```python
from build123d import *

# Parameters (mm, degrees)
F0_W     = 50
F0_H     = 50
F0_W_2   = 46
F0_H_2   = 46
F1_DEPTH = 860
F2_R     = 2.5
F3_R     = 2.5


with BuildPart() as f1:
    # F0 (on Top) → F1 (new body)
    with BuildSketch(Plane.XY):
        with Locations((-29.158926, 36.710037)):
            Rectangle(F0_W, F0_H)
        with Locations((-29.158926, 36.710037)):
            Rectangle(F0_W_2, F0_H_2, mode=Mode.SUBTRACT)
    extrude(amount=F1_DEPTH)

    # F2
    f2_edges = [f1.edges().sort_by_distance(p)[0] for p in [
        (-4.158926, 61.710037, 430),
        (-54.158926, 61.710037, 430),
        (-4.158926, 11.710037, 430),
        (-54.158926, 11.710037, 430),
    ]]
    fillet(f2_edges, radius=F2_R)

    # F3
    f3_edges = [f1.edges().sort_by_distance(p)[0] for p in [
        (-6.158926, 59.710037, 430),
        (-52.158926, 59.710037, 430),
        (-52.158926, 13.710037, 430),
        (-6.158926, 13.710037, 430),
    ]]
    fillet(f3_edges, radius=F3_R)


with BuildPart() as f4_1:
    # F4: copy of F1
    add(f1.part)


with BuildPart() as f6_1:
    # F6: copy of F1
    add(f1.part)


solid = f1.part
```
The model under review builds one solid part; all positions refer to its coordinate system, in mm. A direction names the side the tool comes from. Round coordinates to 2 decimals unless told otherwise and drop trailing zeros. Write each loop counter-clockwise with the first axis right and the second up, starting at its lowest first coordinate (ties: lowest second). Pieces come first, ordered by that corner, then holes.
(1) Machinability: for faces 4 (the flat face through (-29, 61, 0)), 5 (the flat face through (-29, 13.71, 424)), which of the approach directions +Z, -Z, +X, -X, +Y, -Y give a long, thin tool a straight path to every point of the face, cutting with its end or side? Answer none if there is none.
(2) Wall thickness on L1, parallel to Y at x = -40, z = 469; L2, parallel to X at y = 33.5, z = 536; L3, parallel to X at y = 14, z = 528: over which ranges is each line inside the solid? List them lowest first.
(3) We need section C-C on z = 771.5. Give the boundary of the cut face in (x, y).
(4) Mouldability with a two-part tool opening along X and no side actions: class faces 1 (the flat face through (-52.159, 36, 424)), 2 (the flat face through (-29, 61, 860)), 3 (the flat face through (-4.159, 36, 424)) as +X half, -X half, draft (parallel to the pull), parting line (faces both ways), or undercut.
(5) We need section B-B on y = 41. Give the boundary of the cut face in (x, z), and give its area (3 significant figures).
(6) We need section A-A on x = -20.5. Give the boundary of the cut face in (y, z), and give its area (3 significant figures).
Findings below:
1. face 4: -Z, +X, -X, +Y, -Y
1. face 5: +Z, -Z
2. L1: y = 11.71 to 13.71, 59.71 to 61.71
2. L2: x = -54.16 to -52.16, -6.16 to -4.16
2. L3: x = -54.15 to -50.83, -7.49 to -4.17
3. outline: (-54.16, 14.21) arc R2.5 ccw to (-51.66, 11.71) - (-6.66, 11.71) arc R2.5 ccw to (-4.16, 14.21) - (-4.16, 59.21) arc R2.5 ccw to (-6.66, 61.71) - (-51.66, 61.71) arc R2.5 ccw to (-54.16, 59.21) - close; hole (-52.16, 16.21) arc R2.5 ccw to (-49.66, 13.71) - (-8.66, 13.71) arc R2.5 ccw to (-6.16, 16.21) - (-6.16, 57.21) arc R2.5 ccw to (-8.66, 59.71) - (-49.66, 59.71) arc R2.5 ccw to (-52.16, 57.21) - close
4. face 1: undercut
4. face 2: draft
4. face 3: +X half
5. outline: (-54.16, 0) - (-52.16, 0) - (-52.16, 860) - (-54.16, 860) - close; (-6.16, 0) - (-4.16, 0) - (-4.16, 860) - (-6.16, 860) - close
5. area: 3,440 mm2
6. outline: (11.71, 0) - (13.71, 0) - (13.71, 860) - (11.71, 860) - close; (59.71, 0) - (61.71, 0) - (61.71, 860) - (59.71, 860) - close
6. area: 3,440 mm2
